```python
from build123d import *

# Parameters (mm, degrees)
SKETCH_R      = 1.6
PAD_DEPTH     = 7
SKETCH001_R   = 15
SKETCH001_R_2 = 1.6
PAD001_DEPTH  = 2
CHAMFER_SIZE  = 1


with BuildPart() as part:
    # Sketch → Pad (new body)
    with BuildSketch(Plane.XY):
        with BuildLine():
            ThreePointArc((-2.5, 3.122499), (-3.518971, 1.901799), (-3.981855, 0.380567))
            Line((-5.478695, -0.483634), (-3.981855, 0.380567))
            ThreePointArc((-5.478695, -0.483634), (-4.659167, -2.922699), (-2.81991, -4.722087))
            Line((-1.232265, -3.80546), (-2.81991, -4.722087))
            ThreePointArc((-1.232265, -3.80546), (0.117848, -3.998264), (1.454262, -3.726275))
            Line((2.992718, -4.614503), (1.454262, -3.726275))
            ThreePointArc((2.992718, -4.614503), (4.763149, -2.749985), (5.492638, -0.284484))
            Line((3.954108, 0.604177), (5.492638, -0.284484))
            ThreePointArc((3.954108, 0.604177), (3.46401, 2.000159), (2.5, 3.122499))
            Line((2.5, 3.122499), (2.5, 4.898979))
            ThreePointArc((2.5, 4.898979), (0, 5.5), (-2.5, 4.898979))
            Line((-2.5, 3.122499), (-2.5, 4.898979))
        make_face()
        Circle(SKETCH_R, mode=Mode.SUBTRACT)
    extrude(amount=PAD_DEPTH)

    # Sketch001 (on Face14 of Pad) → Pad001 (join)
    with BuildSketch(Plane(origin=(0, 0, 0), x_dir=(1, 0, 0), z_dir=(0, 0, -1))):
        Circle(SKETCH001_R)
        Circle(SKETCH001_R_2, mode=Mode.SUBTRACT)
    extrude(amount=PAD001_DEPTH)

    # Chamfer
    chamfer_edges = [part.edges().sort_by_distance(p)[0] for p in [
        (-2.026088, -4.263773, 7),
        (0.117848, -3.998264, 7),
        (2.22349, -4.170389, 7),
        (4.763149, -2.749985, 7),
        (3.46401, 2.000159, 7),
        (4.723373, 0.159847, 7),
        (2.5, 4.010739, 7),
        (0, 5.5, 7),
        (-2.5, 4.010739, 7),
        (-3.518971, 1.901799, 7),
        (-4.730275, -0.051534, 7),
        (-4.659167, -2.922699, 7),
    ]]
    chamfer(chamfer_edges, length=CHAMFER_SIZE)


solid = part.part
```
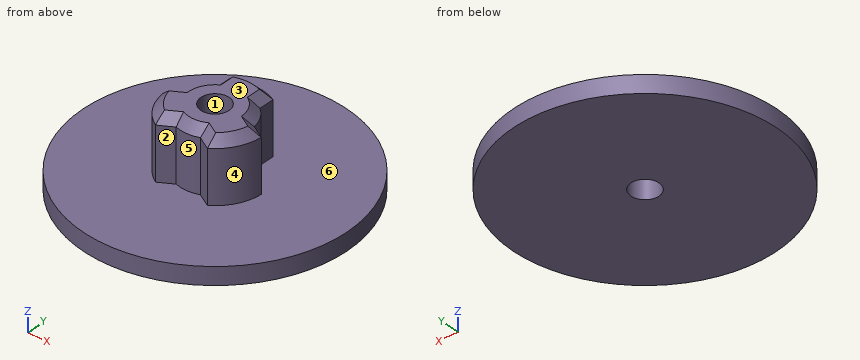
For this review, take the finished solid that the model builds, in its own axes (mm). Face numbers are marked on the shaded views. A direction names the side the tool comes from. Coordinates: 2 decimals unless noted, no trailing zeros. Write each loop counter-clockwise with the first axis right and the second up, starting at its lowest first coordinate (ties: lowest second). Pieces come first, ordered by that corner, then holes. Notation, with made-up numbers: (78.5, 66) - (95.5, 66) arc R24 cw to (95.5, 82) - close; hole circle Ø4 at (40.25, 69.5). An arc over 180 degrees is marked (long way). Put each result on its own line as item: value.
1. Mouldability with a two-part tool opening along Y and no side actions: class the marked faces 1, 2 and 3 as released by +Y, released by -Y, zero draft, split by the parting line, or undercut.
Values found:
face 1: undercut
face 2: released by -Y
face 3: zero draft
2. For pin 1 (5 mm diameter, centred on y = 4, z = 6, fed in from +X); pin 2 (0.9 mm diameter, centred on y = 3.5, z = 4, fed in from +X); pin 3 (1 mm diameter, centred on x = -1, y = -3.5, fed in from +Z); pin 4 (1.9 mm diameter, centred on x = 0, y = 0, fed in from -Z), all flat-tipped, find the tip position at first contact; note any pin that passes through.
Values found:
pin 1: x = 3.71
pin 2: x = 2.59
pin 3: z = 6.86
pin 4: through
3. Add section C-C, the plane y = 7.25. Give the boundary of the cut face in (x, z), then the cut area to 3 significant figures.
Values found:
outline: (-13.13, -2) - (13.13, -2) - (13.13, 0) - (-13.13, 0) - close
area: 52.5 mm²
4. Machinability: for the marked faces 4, 5 and 6, which of the approach directions +Z, -Z, +X, -X, +Y, -Y give a long, thin tool a straight path to every point of the face, cutting with its end or side? Answer none if there is none.
Values found:
face 4: +Z, +X, -Y
face 5: +Z, -Y
face 6: +Z
5. Add section B-B, the plane z = 1. Give the boundary of the cut face in (x, y), then the cut area to 3 significant figures.
Values found:
outline: (-5.48, -0.48) arc R5.5 ccw to (-2.82, -4.72) - (-1.23, -3.81) arc R4 ccw to (1.45, -3.73) - (2.99, -4.61) arc R5.5 ccw to (5.49, -0.28) - (3.95, 0.6) arc R4 ccw to (2.5, 3.12) - (2.5, 4.9) arc R5.5 ccw to (-2.5, 4.9) - (-2.5, 3.12) arc R4 ccw to (-3.98, 0.38) - close; hole circle Ø3.2 at (0, 0)
area: 66.0 mm²
6. Wall thickness on probe 1 along Z at (x, y) = (-5.75, 4); probe 2 along X at (y, z) = (3.5, 1.25); probe 3 along X at (y, z) = (0, 1.75): over which ranges is each line inside the solid? List them lowest first.
Values found:
probe 1: -2 to 0
probe 2: -2.5 to 2.5
probe 3: -4.64 to -1.6, 1.6 to 5
7. Add section A-A, the plane x = 0. Give the boundary of the cut face in (y, z), then the cut area to 3 significant figures.
Values found:
outline: (-15, -2) - (-1.6, -2) - (-1.6, 7) - (-3, 7) - (-4, 6) - (-4, 0) - (-15, 0) - close; (1.6, -2) - (15, -2) - (15, 0) - (5.5, 0) - (5.5, 6) - (4.5, 7) - (1.6, 7) - close
area: 96.7 mm²
8. Add section D-D, the plane x = 11.25. Give the boundary of the cut face in (y, z).
Values found:
outline: (-9.92, -2) - (9.92, -2) - (9.92, 0) - (-9.92, 0) - close
